The model under review builds one solid part; all positions refer to its coordinate system, in mm. Face numbers are marked on the shaded views. Coordinates: 2 decimals unless noted, no trailing zeros. Order: outer loops, then holes, each group sorted by start corner. A loop starts at its lowest first (then second) coordinate and runs counter-clockwise, first axis right, second up. Notation, with made-up numbers: (6, 9.25) -> (65, 9.25) arc R15 ccw to (65, 37.25) -> close; hole circle Ø3 at (-1.75, 48). An arc over 180 degrees is marked (long way). Use one line per item in the form item = value.
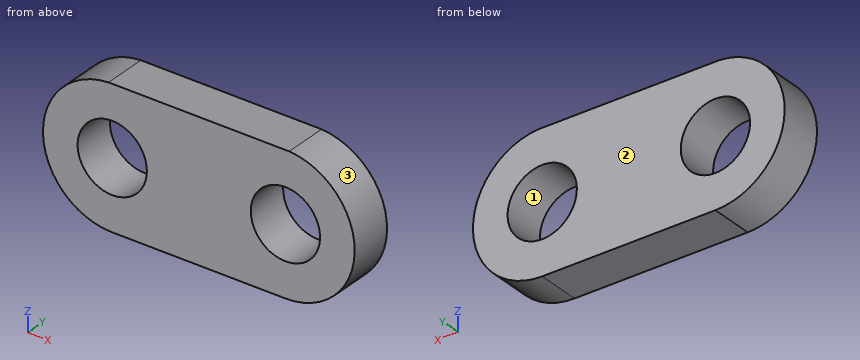
from build123d import *

# Parameters (mm, degrees)
F0_R     = 2
F1_DEPTH = 2.5


with BuildPart() as f1:
    # F0 (on Front) → F1 (new body)
    with BuildSketch(Plane.XZ):
        with BuildLine():
            Line((5.398431, 3.994088), (-4.166759, 3.994088))
            Line((-4.166759, 3.994088), (-4.601569, 3.994088))
            ThreePointArc((-4.601569, 3.994088), (-8.38304, -0.094824), (-4.41201, -3.999903))
            ThreePointArc((-4.41201, -3.999903), (-4.384203, -4), (-4.356396, -3.999904))
            Line((-4.356396, -3.999904), (5.615797, -4))
            ThreePointArc((5.615797, -4), (9.614357, -0.108762), (5.833241, 3.994088))
            Line((5.833241, 3.994088), (5.398431, 3.994088))
        make_face()
        with Locations((-4.384164, 0)):
            Circle(F0_R, mode=Mode.SUBTRACT)
        with BuildLine():
            ThreePointArc((7.615836, 0), (5.615836, -2), (3.615836, 0))
            ThreePointArc((3.615836, 0), (5.615836, 2), (7.615836, 0))
        make_face(mode=Mode.SUBTRACT)
    extrude(amount=F1_DEPTH)


solid = f1.part
Item 1: Clearance check with flat-ended pins moving along their axes: pin 1 (1.5 mm diameter, centred on y = -2, z = 0.5, fed in from +X); pin 2 (1.5 mm diameter, centred on y = -2, z = -2.5, fed in from -X). State where each tip first meets the part, or that it passes through.
Results found:
pin_1 = 9.62
pin_2 = -7.98
Item 2: We need section A-A (z = 0). Write out the cut boundary in (x, y).
Results found:
outline = (-8.38, -2.5) -> (-6.38, -2.5) -> (-6.38, 0) -> (-8.38, 0) -> close; (-2.38, -2.5) -> (3.62, -2.5) -> (3.62, 0) -> (-2.38, 0) -> close; (7.62, -2.5) -> (9.62, -2.5) -> (9.62, 0) -> (7.62, 0) -> close
Item 3: We need section C-C (y = -2.05). Write out the cut boundary in (x, z).
Results found:
outline = (-4.6, 3.99) arc R4 ccw to (-4.41, -4) arc R4.01 ccw to (-4.36, -4) -> (5.62, -4) arc R4 ccw to (5.83, 3.99) -> close; hole circle Ø4 at (-4.38, 0); hole circle Ø4 at (5.62, 0)
Item 4: We need section D-D (x = -5.25). Write out the cut boundary in (y, z).
Results found:
outline = (-2.5, -3.91) -> (0, -3.91) -> (0, -1.8) -> (-2.5, -1.8) -> close; (-2.5, 1.8) -> (0, 1.8) -> (0, 3.91) -> (-2.5, 3.91) -> close
Item 5: To check wall thickness, follow L1, parallel to Z at x = 5.75, y = -0.15; L2, parallel to X at y = -1.7, z = 1.25; L3, parallel to X at y = -0.4, z = -0.25. State the ranges of each line that lie inside material, in increasing order. Write a range as from..to.
Results found:
L1 = -4..-2, 2..3.99
L2 = -8.18..-5.95, -2.82..4.05, 7.18..9.42
L3 = -8.38..-6.37, -2.4..3.63, 7.6..9.61
Item 6: Draft analysis for pull direction X (two halves, no side actions). For the marked faces 1, 2 and 3, state which applies: released by +X, released by -X, zero draft, split by the parting line, or undercut.
Results found:
face_1 = undercut
face_2 = zero draft
face_3 = released by +X
Item 7: We need section B-B (x = -3). Write out the cut boundary in (y, z).
Results found:
outline = (-2.5, -4) -> (0, -4) -> (0, -1.44) -> (-2.5, -1.44) -> close; (-2.5, 1.44) -> (0, 1.44) -> (0, 3.99) -> (-2.5, 3.99) -> close
